Can you work these out from the model? Positions are in its coordinate system, mm. A direction names the side the tool comes from. Give positions to 0.01 mm unless a question says otherwise; leave off trailing zeros. Write each loop counter-clockwise with the first axis right and the second up, starting at its lowest first coordinate (ties: lowest second). Pieces come first, ordered by that corner, then holes.
```python
from build123d import *

# Parameters (mm, degrees)
SKETCH1_W           = 88.9
SKETCH1_H           = 12.7
BOSS_EXTRUDE1_DEPTH = 2.54
FILLET1_R           = 0.635
SHELL1_START        = 0.635
SHELL1_OUTLINE_W    = 1.905
SHELL1_OUTLINE_H    = 11.43
SHELL1_DEPTH        = 87.63
SKETCH2_R           = 2.54
BOSS_EXTRUDE2_DEPTH = 2.54


# Read off the part's stored shape, not the designer's step: Shell1
with BuildPart() as part:
    # Sketch1 → Boss-Extrude1 (new body)
    with BuildSketch(Plane(origin=(0, 0, 0), x_dir=(1, 0, 0), z_dir=(0, 1, 0))):
        with Locations((44.45, 6.35)):
            Rectangle(SKETCH1_W, SKETCH1_H)
    extrude(amount=BOSS_EXTRUDE1_DEPTH)

    # Fillet1
    fillet1_edges = [part.edges().sort_by_distance(p)[0] for p in [
        (0, 1.27, -12.7),
        (88.9, 1.27, -12.7),
        (88.9, 1.27, 0),
        (0, 1.27, 0),
    ]]
    fillet(fillet1_edges, radius=FILLET1_R)

    # Shell1 outline → Shell1 (cut)
    with BuildSketch(Plane.YZ.offset(SHELL1_START)):
        with Locations((0.9525, -6.35)):
            Rectangle(SHELL1_OUTLINE_W, SHELL1_OUTLINE_H)
    extrude(amount=SHELL1_DEPTH, mode=Mode.SUBTRACT)

    # Sketch2 → Boss-Extrude2 (add)
    with BuildSketch(Plane(origin=(0, 1.905, 0), x_dir=(-1, 0, 0), z_dir=(0, -1, 0))):
        with Locations(Location((-69.85, 6.35, 0), (0, 0, 270))):
            Circle(SKETCH2_R)
        with Locations(Location((-19.05, 6.35, 0), (0, 0, 270))):
            Circle(SKETCH2_R)
    extrude(amount=BOSS_EXTRUDE2_DEPTH)


solid = part.part
```
1) Suppose I cut it at C-C on z = -6.35. Write out the boundary of the cut face in (x, y) (3 decimals), plus the area to 3 significant figures.
Values follow:
outline: (0, 0) - (0.635, 0) - (0.635, 1.905) - (16.51, 1.905) - (16.51, -0.635) - (21.59, -0.635) - (21.59, 1.905) - (67.31, 1.905) - (67.31, -0.635) - (72.39, -0.635) - (72.39, 1.905) - (88.265, 1.905) - (88.265, 0) - (88.9, 0) - (88.9, 2.54) - (0, 2.54) - close
area: 84.7 mm2
2) Suppose I cut it at B-B on x = 19.05. Write out the boundary of the cut face in (y, z) (3 decimals), plus the area to 3 significant figures.
Values follow:
outline: (-0.635, -8.89) - (1.905, -8.89) - (1.905, -12.065) - (0, -12.065) - (0, -12.7) - (2.54, -12.7) - (2.54, 0) - (0, 0) - (0, -0.635) - (1.905, -0.635) - (1.905, -3.81) - (-0.635, -3.81) - close
area: 23.4 mm2
3) If we mould it in two halves opening along X, with no side actions, what happens to faces 3 (the face through (0, 1, -6)), 4 (the face through (44.2, 0, -0.3)), 5 (the face through (44, 1, -12.065))? For each: +X half, -X half, draft (parallel to the pull), parting line (faces both ways), or undercut.
Values follow:
face 3: -X half
face 4: draft
face 5: undercut
4) Suppose I cut it at A-A on y = 0.6. Write out the boundary of the cut face in (x, z) (3 decimals).
Values follow:
outline: (0, -12.065) arc R0.635 ccw to (0.635, -12.7) - (88.265, -12.7) arc R0.635 ccw to (88.9, -12.065) - (88.9, -0.635) arc R0.635 ccw to (88.265, 0) - (0.635, 0) arc R0.635 ccw to (0, -0.635) - close; circle Ø5.08 at (19.05, -6.35); circle Ø5.08 at (69.85, -6.35); hole (0.635, -12.065) - (88.265, -12.065) - (88.265, -0.635) - (0.635, -0.635) - close
5) Suppose I cut it at D-D on x = 78.5. Write out the boundary of the cut face in (y, z) (3 decimals).
Values follow:
outline: (0, -12.7) - (2.54, -12.7) - (2.54, 0) - (0, 0) - (0, -0.635) - (1.905, -0.635) - (1.905, -12.065) - (0, -12.065) - close
6) For pin 1 Ø5.5 at (x, z) = (52.5, -4) entering from -Y (3 decimals), with a flat end and sliding along its axis, tell me the tip position at first contact or that it passes through.
Values follow:
pin 1: stops at y = 1.905
7) For faces 1 (the face through (70, -0.635, -6)), 2 (the face through (0.635, 1, -6)), which set-ups out of +Z, -Z, +X, -X, +Y, -Y let a thin tool reach every point of the face, with its end or its side?
Values follow:
face 1: +Z, -Z, +X, -X, -Y
face 2: -Y
8) Please list where these lines run through material, in increasing order: L1, parallel to X at y = 1.8, z = -10.25 (3 decimals); L2, parallel to Z at x = 66.5, y = 0.3 (3 decimals); L3, parallel to X at y = 0.7, z = -5.5 (3 decimals).
Values follow:
L1: x = 0 to 0.635, 88.265 to 88.9
L2: z = -12.7 to -12.065, -0.635 to 0
L3: x = 0 to 0.635, 16.656 to 21.444, 67.456 to 72.244, 88.265 to 88.9
